from build123d import *

# Parameters (mm, degrees)
CUT_EXTRUDE_START   = -12
CUT_EXTRUDE_1_DEPTH = 12
CUT_EXTRUDE_START_2 = -13.5
SKETCH_3_R          = 3
CUT_EXTRUDE_2_DEPTH = 13.5


with BuildPart() as part:
    # ｽｹｯﾁ1 → 回転1 (revolve)
    with BuildSketch(Plane.XY, mode=Mode.PRIVATE) as revolve_1_sk:
        Polygon((0, 0), (0, 42.3), (3, 42.3), (3, 15.05), (5.05, 15.05), (5.05, 13.9), (10.225, 13.9), (10.225, 9.9), (3, 9.9), (3, 4.45), (2, 3.45), (1.25, 3.45), (1.25, 0), align=None)
    revolve(revolve_1_sk.sketch.rotate(Axis((0, 0, 0), (0, 1, 0)), 90), axis=Axis((0, 0, 0), (0, 1, 0)))

    # ｽｹｯﾁ2 → ｶｯﾄ - 押し出し1 (cut)
    with BuildSketch(Plane(origin=(0, 42.3, 0), x_dir=(1, 0, 0), z_dir=(0, 1, 0)).offset(CUT_EXTRUDE_START)):
        with BuildLine():
            Line((-1.658312395, 2.5), (1.658312395, 2.5))
            ThreePointArc((1.658312395, 2.5), (0, 3), (-1.658312395, 2.5))
        make_face()
    extrude(amount=CUT_EXTRUDE_1_DEPTH, mode=Mode.SUBTRACT)

    # ｽｹｯﾁ3 → ｶｯﾄ - 押し出し2 (cut)
    with BuildSketch(Plane(origin=(0, 42.3, 0), x_dir=(1, 0, 0), z_dir=(0, 1, 0)).offset(CUT_EXTRUDE_START_2)):
        with Locations(Location((0, 0, 0), (0, 0, 90))):
            Circle(SKETCH_3_R)
    extrude(amount=CUT_EXTRUDE_2_DEPTH, mode=Mode.SUBTRACT)


solid = part.part
Verification items for the finished model (mm, model axes). A direction names the side the tool comes from. Round coordinates to 2 decimals unless told otherwise and drop trailing zeros. Loops run counter-clockwise (first coordinate to the right, second up) from the corner with the lowest first, then second, coordinate; pieces in that order, holes last. Notation, with made-up numbers: (-25, -22.75) - (-15, -22.75) arc R15 cw to (-15, -8.75) - close; hole circle Ø2 at (-37, 18.5). An arc over 180 degrees is marked (long way). Answer in a Markdown table with one row per item. Add a question column.
Q1. Gauge pin test, flat ends, axial feed: pin 1 (10 mm diameter, centred on y = 4, z = -1, fed in from +X); pin 2 (4 mm diameter, centred on y = 6.5, z = -4, fed in from +X); pin 3 (1.5 mm diameter, centred on x = 4.5, z = 5, fed in from -Y); pin 4 (6 mm diameter, centred on y = 17, z = -7.5, fed in from -X). Record the tip position at first contact, or that the pin passes through.
Q2. Tool access check on faces 1 (the face through (2, 13.9, -5)), 2 (the face through (0, 28.8, 0)), 3 (the face through (-0.05, 1.7, 1.25)). Record the directions out of +Z, -Z, +X, -X, +Y, -Y that give a thin tool (end or side, any length) a straight path to the whole face; none if there is none.
Q3. Section check D-D on y = 2.25. Enter the section's corners in (x, z), plus the area to 3 significant figures.
Q4. Section check B-B on z = 0. Enter the section's corners in (x, y) (3 decimals), plus the area to 3 significant figures.
Q5. Material ranges on line 1 (Y direction, x = -5, z = -4.5); line 2 (Y direction, x = -2, z = -2.5); line 3 (X direction, y = 1.5, z = 0.25), recorded low to high.
Q6. Section check C-C on y = 11. Enter the section's corners in (x, z) (3 decimals).
Q7. Section check A-A on x = 0. Enter the section's corners in (y, z) (3 decimals).
Found:
| question | item | result |
|---|---|---|
| 1 | pin 1 | stops at x = 3 |
| 1 | pin 2 | stops at x = 2.24 |
| 1 | pin 3 | stops at y = 9.9 |
| 1 | pin 4 | passes through |
| 2 | face 1 | +Y |
| 2 | face 2 | +Z, -Z, +X, -X, +Y |
| 2 | face 3 | -Y |
| 3 | outline | circle Ø2.5 at (0, 0) |
| 3 | area | 4.91 mm² |
| 4 | outline | (-10.225, 9.9) - (-3, 9.9) - (-3, 4.45) - (-2, 3.45) - (-1.25, 3.45) - (-1.25, 0) - (1.25, 0) - (1.25, 3.45) - (2, 3.45) - (3, 4.45) - (3, 9.9) - (10.225, 9.9) - (10.225, 13.9) - (5.05, 13.9) - (5.05, 15.05) - (3, 15.05) - (3, 28.8) - (-3, 28.8) - (-3, 15.05) - (-5.05, 15.05) - (-5.05, 13.9) - (-10.225, 13.9) - close |
| 4 | area | 222 mm² |
| 5 | line 1 | y = 9.9 to 13.9 |
| 5 | line 2 | y = 9.9 to 15.05 |
| 5 | line 3 | x = -1.22 to 1.22 |
| 6 | outline | circle Ø20.45 at (0, 0) |
| 7 | outline | (0, -1.25) - (3.45, -1.25) - (3.45, -2) - (4.45, -3) - (9.9, -3) - (9.9, -10.225) - (13.9, -10.225) - (13.9, -5.05) - (15.05, -5.05) - (15.05, -3) - (28.8, -3) - (28.8, 3) - (15.05, 3) - (15.05, 5.05) - (13.9, 5.05) - (13.9, 10.225) - (9.9, 10.225) - (9.9, 3) - (4.45, 3) - (3.45, 2) - (3.45, 1.25) - (0, 1.25) - close |
